Design review of the part built by this model. Coordinates are the model's own, in mm. A direction names the side the tool comes from. Coordinates: 2 decimals unless noted, no trailing zeros. Loops run counter-clockwise (first coordinate to the right, second up) from the corner with the lowest first, then second, coordinate; pieces in that order, holes last. Notation, with made-up numbers: (87.25, 12) -> (108.25, 12) arc R18 cw to (108.25, 39) -> close; hole circle Ø5 at (-6, -28). An arc over 180 degrees is marked (long way). Use one line per item in the form item = value. Start each with the question number.
1. Machinability: for faces 1 (the face through (0, 14, 32)), 2 (the face through (0, -13, 33)), 3 (the face through (1.521, -14.504, -31.962)), which of the approach directions +Z, -Z, +X, -X, +Y, -Y give a long, thin tool a straight path to every point of the face, cutting with its end or side? Answer none if there is none.
2. Consider section B-B (z = 33). State how many separate pieces and enclosed holes the cut face has, then the cut area to 3 significant figures.
3. Consider section C-C (y = 16.5). State the section outline as (x, z) points, then the cut area to 3 significant figures.
4. For pin 1 (4 mm diameter, centred on x = -10, z = -5.5, fed in from -Y); pin 2 (1 mm diameter, centred on x = 0.5, z = 6.5, fed in from +Y); pin 3 (6 mm diameter, centred on y = 11.5, z = -30, fed in from -X), all flat-tipped, find the tip position at first contact; note any pin that passes through.
5. The part is to be moulded in two halves that separate along Z. For faces 4 (the face through (2, 15, -27)), 5 (the face through (-1.6, -0.3, 39)), 6 (the face through (0, 14, -34)), say which applies: released by +Z, released by -Z, zero draft, split by the parting line, or undercut.
6. Wall thickness on line 1 (Y direction, x = 2, z = 33); line 2 (Z direction, x = 1.5, y = 13); line 3 (Z direction, x = 1.2, y = -16.5): over which ranges is each line inside the solid? List them lowest first. Write a range as from..to.
7. Consider section A-A (y = -10.5). State the section outline as (x, z) points, then the cut area to 3 significant figures.
Autodesk Inventor part; units mm, degrees
ref_plane "YZ Plane" through (0, 0, 0) normal (1, 0, 0) x (0, 1, 0)
ref_plane "XZ Plane" through (0, 0, 0) normal (0, 1, 0) x (-1, 0, 0)
ref_plane "XY Plane" through (0, 0, 0) normal (0, 0, 1) x (1, 0, 0)
sketch "Sketch1" plane through (0, 0, 0) normal (1, 0, 0) x (0, 1, 0)
  line L0 (-22.5, 39) -> (22.5, 39)
  line L1 (22.5, -39) -> (-22.5, -39)
  line L2 (-22.5, 39) -> (22.5, -39) construction
  line L3 (22.5, 39) -> (-22.5, -39) construction
  line L4 (22.5, 39) -> (22.5, -39)
  line L5 (-22.5, -39) -> (-22.5, 39)
  line L6 (22.5, 0) -> (-22.5, 0)
  point P0 (0, 0)
  point P1 (16.5, 33)
  point P2 (-16.5, 33)
  point P3 (16.5, -33)
  point P4 (-16.5, -33)
  dimension "d43" = 78
  dimension "d44" = 45
  dimension "d45" = 6
  dimension "d46" = 6
  dimension "d47" = 6
  dimension "d48" = 6
extrude "Extrusion3" add sketch "Sketch1" along normal blind 3
hole "Hole3" at (0, 16.5, 33) at (0, 16.5, -33) at (0, -16.5, -33) at (0, -16.5, 33) direction (1, 0, 0) diameter 4.5 end through all
sketch "Sketch4" plane through (0, 0, 0) normal (-1, 0, 0) x (0, 0, 1)
  line L0 (39, 22.5) -> (39, -22.5)
  line L1 (-39, -6.5) -> (39, -6.5)
  line L2 (39, -6.5) -> (39, 6.5)
  line L3 (39, 6.5) -> (-39, 6.5)
  line L4 (-39, 6.5) -> (-39, -6.5)
  line L5 (-39, -6.5) -> (39, 6.5) construction
  line L6 (39, -6.5) -> (-39, 6.5) construction
  point P0 (0, 0)
  dimension "d49" = 13
extrude "Extrusion4" add sketch "Sketch4" along normal blind 13
full round fillet "Full Round Fillet2" first side at (-4.3333, -6.5, -13) centre faces at (-13, 2.1667, -13) second side at (-4.3333, 6.5, 13)
sketch "Sketch5" plane through (0, -22.5, 39) normal (0, 0, 1) x (1, 0, 0)
  line L0 (0, 29) -> (-6.5, 29)
  point P0 (0, 22.5)
  point P1 (-6, 22.5)
  dimension "d52" = 6
  dimension "d53" = 6.5
hole "Hole4" at (-6, 0, 39) direction (0, 0, -1) diameter 8 end through all
sketch "Sketch6" plane through (3, 0, 0) normal (1, 0, 0) x (0, 0, -1)
  line L0 (39, 22.5) -> (-39, 22.5)
  line L1 (39, 6.5) -> (-39, 6.5)
  line L2 (-27, 22.5) -> (27, 22.5)
  line L3 (27, 22.5) -> (27, 6.5)
  line L4 (27, 6.5) -> (-27, 6.5)
  line L5 (-27, 6.5) -> (-27, 22.5)
  line L6 (-39, -22.5) -> (39, -22.5)
  line L7 (-27, -22.5) -> (27, -22.5)
  line L8 (27, -22.5) -> (27, -6.5)
  line L9 (27, -6.5) -> (-27, -6.5)
  line L10 (-27, -6.5) -> (-27, -22.5)
  line L11 (-39, -6.5) -> (39, -6.5)
  circle A0 centre (33, 16.5) radius 2.25
  circle A1 centre (-33, 16.5) radius 2.25
  point P0 (0, 0)
  point P1 (27, -22.5)
  dimension "d61" = 0
  dimension "d62" = 6
  dimension "d63" = 6
extrude "Extrusion5" cut sketch "Sketch6" against normal blind 10 contours L3 L1 L5 L0 | L10 L9 L8 L6
properties part number "Axle Hold"
Geometry check:
q1.face_1 = +Z, -Z, -X, +Y
q1.face_2 = +Z, -Z, -X, -Y
q1.face_3 = +X, -X
q2.separate_pieces = 3
q2.enclosed_holes = 1
q2.area = 209 mm²
q3.outline = (0, -39) -> (3, -39) -> (3, -35.25) -> (0, -35.25) -> close; (0, -30.75) -> (3, -30.75) -> (3, -27) -> (0, -27) -> close; (0, 27) -> (3, 27) -> (3, 30.75) -> (0, 30.75) -> close; (0, 35.25) -> (3, 35.25) -> (3, 39) -> (0, 39) -> close
q3.area = 45.0 mm²
q4.pin_1 = -6.32
q4.pin_2 = 6.5
q4.pin_3 = 0
q5.face_4 = undercut
q5.face_5 = released by +Z
q5.face_6 = zero draft
q6.line_1 = -22.5..-18.75, -14.25..14.25, 18.75..22.5
q6.line_2 = -39..-27, 27..39
q6.line_3 = -39..-35.25, -30.75..-27, 27..30.75, 35.25..39
q7.outline = (0, -39) -> (3, -39) -> (3, -27) -> (0, -27) -> close; (0, 27) -> (3, 27) -> (3, 39) -> (0, 39) -> close
q7.area = 72.0 mm²
